from build123d import *

# Parameters (mm, degrees)
SKETCH1_W           = 50
SKETCH1_H           = 49.309999932
BOSS_EXTRUDE1_DEPTH = 22.098
SKETCH11_R          = 1.5875
CUT_EXTRUDE7_DEPTH  = 33.02
CUT_EXTRUDE8_DEPTH  = 2.54
BOSS_EXTRUDE5_DEPTH = 2.54
BOSS_EXTRUDE6_DEPTH = 7.5
SKETCH14_R          = 1.5875
SKETCH14_W          = 12.7
SKETCH14_H          = 12.7
CUT_EXTRUDE9_DEPTH  = 2.54
SKETCH20_W          = 6
SKETCH20_H          = 6.5
CUT_EXTRUDE13_DEPTH = 7.5
SKETCH22_R          = 2.667
BOSS_EXTRUDE7_DEPTH = 13.97999998
SKETCH24_R          = 1.5875
BOSS_EXTRUDE9_DEPTH = 2.54


with BuildPart() as part:
    # Sketch1 → Boss-Extrude1 (new body)
    with BuildSketch(Plane.XY):
        with Locations((0, 0.745000034)):
            Rectangle(SKETCH1_W, SKETCH1_H)
        Polygon((12.5, 47.050635095), (-12.5, 47.050635095), (-25, 25.4), (25, 25.4), align=None)
    extrude(amount=BOSS_EXTRUDE1_DEPTH)

    # Sketch11 → Cut-Extrude7 (cut)
    with BuildSketch(Plane.XY.offset(22.098)):
        with BuildLine():
            Line((-18.015, 22.179409051), (-19.92, 22.179409051))
            Line((-19.92, 22.179409051), (-19.92, -11.209999932))
            Line((-19.92, -11.209999932), (-18.65, -11.209999932))
            ThreePointArc((-18.65, -11.209999932), (-14.159871939, -13.069871871), (-12.3, -17.559999932))
            Line((-12.3, -17.559999932), (-12.3, -18.829999932))
            Line((-12.3, -18.829999932), (12.3, -18.829999932))
            Line((12.3, -18.829999932), (12.3, -17.559999932))
            ThreePointArc((12.3, -17.559999932), (14.159871939, -13.069871871), (18.65, -11.209999932))
            Line((18.65, -11.209999932), (19.92, -11.209999932))
            Line((19.92, -11.209999932), (19.92, 24.038818102))
            Line((19.92, 24.038818102), (18.060590949, 27.259409051))
            Line((18.060590949, 27.259409051), (9.567060633, 41.970635095))
            Line((9.567060633, 41.970635095), (-9.567060633, 41.970635095))
            Line((-9.567060633, 41.970635095), (-18.060590949, 27.259409051))
            Line((-18.060590949, 27.259409051), (-18.015, 27.259409051))
            ThreePointArc((-18.015, 27.259409051), (-12.935, 24.719409051), (-18.015, 22.179409051))
        make_face()
        with Locations((-16.11, 24.719409051)):
            Circle(SKETCH11_R)
        with Locations((16.11, -15.02)):
            Circle(SKETCH11_R)
        with Locations((-16.11, -15.02)):
            Circle(SKETCH11_R)
    extrude(amount=-CUT_EXTRUDE7_DEPTH, mode=Mode.SUBTRACT)

    # Sketch12 → Cut-Extrude8 (cut)
    with BuildSketch(Plane(origin=(0, 0, 0), x_dir=(-1, 0, 0), z_dir=(0, 0, -1))):
        Polygon((-22.46, 25.4), (-22.46, -21.369999932), (22.46, -21.369999932), (22.46, 25.4), (11.23, 44.850930569), (-11.23, 44.850930569), align=None)
    extrude(amount=-CUT_EXTRUDE8_DEPTH, mode=Mode.SUBTRACT)

    # Sketch13 → Boss-Extrude5 (add)
    with BuildSketch(Plane.XY.offset(22.098)):
        Polygon((-25, 25.4), (-25, -23.909999932), (25, -23.909999932), (25, 25.4), (12.5, 47.050635095), (-12.5, 47.050635095), align=None)
    extrude(amount=-BOSS_EXTRUDE5_DEPTH)

    # Sketch19 → Boss-Extrude6 (add)
    with BuildSketch(Plane(origin=(0, 0, 19.558), x_dir=(-1, 0, 0), z_dir=(0, 0, -1))):
        Polygon((-11.968279908, 28.961226002), (-11.968279908, 24.921226002), (-9.698279908, 24.921226002), (-9.698279908, 26.191226002), (-10.698279908, 26.191226002), (-10.698279908, 27.691226002), (-9.698279908, 27.691226002), (-9.698279908, 28.961226002), align=None)
        Polygon((4.601720092, 27.691226002), (4.601720092, 26.191226002), (3.601720092, 26.191226002), (3.601720092, 24.921226002), (5.871720092, 24.921226002), (5.871720092, 28.961226002), (3.601720092, 28.961226002), (3.601720092, 27.691226002), align=None)
    extrude(amount=BOSS_EXTRUDE6_DEPTH)

    # Sketch14 → Cut-Extrude9 (cut)
    with BuildSketch(Plane(origin=(0, 0, 19.558), x_dir=(-1, 0, 0), z_dir=(0, 0, -1))):
        with Locations((-10.16, 6.35)):
            Circle(SKETCH14_R)
        with Locations((10.16, 6.35)):
            Circle(SKETCH14_R)
        with Locations((10.16, -6.35)):
            Circle(SKETCH14_R)
        with Locations((-10.16, -6.35)):
            Circle(SKETCH14_R)
        Rectangle(SKETCH14_W, SKETCH14_H)
    extrude(amount=-CUT_EXTRUDE9_DEPTH, mode=Mode.SUBTRACT)

    # Sketch20 → Cut-Extrude13 (cut)
    with BuildSketch(Plane(origin=(0, 0, 19.558), x_dir=(-1, 0, 0), z_dir=(0, 0, -1))):
        with Locations((-0.698279908, 30.191226002)):
            Rectangle(SKETCH20_W, SKETCH20_H)
    extrude(amount=-CUT_EXTRUDE13_DEPTH, mode=Mode.SUBTRACT)

    # Sketch22 → Boss-Extrude7 (add)
    with BuildSketch(Plane.XY.offset(22.098)):
        with BuildLine():
            Line((26.155685571, 27.78125), (23.625184671, 27.78125))
            Line((23.625184671, 27.78125), (25, 25.4))
            Line((25, 25.4), (25, 23.33625))
            Line((25, 23.33625), (30.600685571, 23.33625))
            ThreePointArc((30.600685571, 23.33625), (33.743775214, 30.924339642), (26.155685571, 27.78125))
        make_face()
        with Locations((30.600685571, 27.78125)):
            Circle(SKETCH22_R, mode=Mode.SUBTRACT)
    extrude(amount=-BOSS_EXTRUDE7_DEPTH)

    # Sketch24 → Boss-Extrude9 (add)
    with BuildSketch(Plane(origin=(0, 0, 2.54), x_dir=(-1, 0, 0), z_dir=(0, 0, -1))):
        Polygon((11.23, 44.850930569), (-11.23, 44.850930569), (-22.46, 25.4), (-22.46, -21.369999932), (22.46, -21.369999932), (22.46, 25.4), align=None)
        with Locations(Location((16.11, -15.02, 0), (0, 0, 180))):
            Circle(SKETCH24_R, mode=Mode.SUBTRACT)
        with Locations(Location((16.11, 24.719409051, 0), (0, 0, 180))):
            Circle(SKETCH24_R, mode=Mode.SUBTRACT)
        with Locations(Location((-16.11, -15.02, 0), (0, 0, 180))):
            Circle(SKETCH24_R, mode=Mode.SUBTRACT)
        with BuildLine():
            Line((-19.92, 24.038818102), (-9.567060633, 41.970635095))
            Line((-9.567060633, 41.970635095), (9.567060633, 41.970635095))
            Line((9.567060633, 41.970635095), (18.060590949, 27.259409051))
            Line((18.060590949, 27.259409051), (18.015, 27.259409051))
            ThreePointArc((18.015, 27.259409051), (12.935, 24.719409051), (18.015, 22.179409051))
            Line((18.015, 22.179409051), (19.92, 22.179409051))
            Line((19.92, 22.179409051), (19.92, -11.209999932))
            Line((19.92, -11.209999932), (18.65, -11.209999932))
            ThreePointArc((18.65, -11.209999932), (14.159871939, -13.069871871), (12.3, -17.559999932))
            Line((12.3, -17.559999932), (12.3, -18.829999932))
            Line((12.3, -18.829999932), (-12.3, -18.829999932))
            Line((-12.3, -18.829999932), (-12.3, -17.559999932))
            ThreePointArc((-12.3, -17.559999932), (-14.159871939, -13.069871871), (-18.65, -11.209999932))
            Line((-18.65, -11.209999932), (-19.92, -11.209999932))
            Line((-19.92, -11.209999932), (-19.92, 24.038818102))
        make_face(mode=Mode.SUBTRACT)
    extrude(amount=BOSS_EXTRUDE9_DEPTH)


solid = part.part
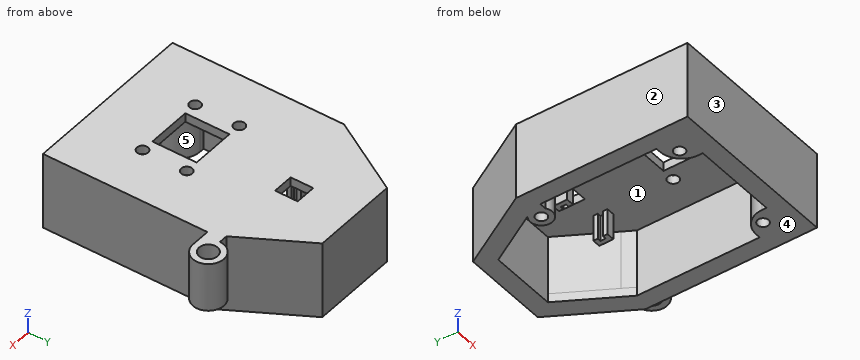
Work out the finished part from the listing and answer in its coordinate system (mm). Face numbers are marked on the shaded views. A direction names the side the tool comes from. Give positions to 0.01 mm unless a question says otherwise; leave off trailing zeros. Order: outer loops, then holes, each group sorted by start corner. A loop starts at its lowest first (then second) coordinate and runs counter-clockwise, first axis right, second up. Notation, with made-up numbers: (57, 26) -> (83, 26) arc R23 cw to (83, 39) -> close; hole circle Ø10 at (47, -17). An arc over 180 degrees is marked (long way). One line per item, written item: value.
Item 1: Find section B-B, the plane y = 18. Give the vertices of the cut face in (x, z), plus the area to 3 significant figures.
Answer sheet:
outline: (-25, 0) -> (-19.92, 0) -> (-19.92, 19.56) -> (19.92, 19.56) -> (19.92, 0) -> (25, 0) -> (25, 22.1) -> (-25, 22.1) -> close
area: 326 mm²
Item 2: Find section C-C, the plane z = 6.75. State how many separate pieces and enclosed holes the cut face has, plus the area to 3 significant figures.
Answer sheet:
separate pieces: 1
enclosed holes: 4
area: 1,150 mm²
Item 3: A tool of negligible diameter and unlimited length cuts with its end or side. For the marked faces 4 and 5, from which of +Z, -Z, +X, -X, +Y, -Y can it reach the whole face along a straight path? Write none if from no direction.
Answer sheet:
face 4: -Z, +X, -X, +Y, -Y
face 5: -Z
Item 4: Straight lines are drawn through the part: probe 1 along Y at (x, z) = (10.16, 20.55); probe 2 along X at (y, z) = (18.5, 10.5); probe 3 along Y at (x, z) = (-16.11, 10.5). For each, find the intervals that lie inside material, in ascending order.
Answer sheet:
probe 1: -23.91 to -7.94, -4.76 to 4.76, 7.94 to 47.05
probe 2: -25 to -19.92, 19.92 to 25
probe 3: -23.91 to -16.61, -13.43 to -11.74, 21.54 to 23.13, 26.31 to 27.89, 30.64 to 40.8
Item 5: Determine the mould class of the marked faces 1, 2 and 3 for opening direction X: released by +X, released by -X, zero draft, split by the parting line, or undercut.
Answer sheet:
face 1: undercut
face 2: released by -X
face 3: zero draft
Item 6: Flat-ended cylindrical pins translate along their axes: P1, Ø1, axis at x = 7.5, y = 25, coming from the -Z side; P2, Ø1.2, axis at y = 26.5, z = 14.5, coming from the -X side; P3, Ø2, axis at x = 25, z = 17.5, coming from the +Y side; P4, Ø1.4, axis at y = 28.5, z = 17, coming from the +X side. Find the tip coordinate at first contact, or state that the pin passes through.
Answer sheet:
P1: z = 19.56
P2: x = -24.71
P3: y = 27.78
P4: x = 35.05
Item 7: Find section A-A, the plane y = 3. Give the vertices of the cut face in (x, z).
Answer sheet:
outline: (-25, 0) -> (-19.92, 0) -> (-19.92, 19.56) -> (-6.35, 19.56) -> (-6.35, 22.1) -> (-25, 22.1) -> close; (6.35, 19.56) -> (19.92, 19.56) -> (19.92, 0) -> (25, 0) -> (25, 22.1) -> (6.35, 22.1) -> close
Item 8: Find section D-D, the plane x = -16.11. Give the vertices of the cut face in (y, z).
Answer sheet:
outline: (-23.91, 0) -> (-16.61, 0) -> (-16.61, 19.56) -> (-13.43, 19.56) -> (-13.43, 0) -> (-11.74, 0) -> (-11.74, 19.56) -> (21.54, 19.56) -> (21.54, 0) -> (23.13, 0) -> (23.13, 19.56) -> (26.31, 19.56) -> (26.31, 0) -> (27.89, 0) -> (27.89, 19.56) -> (30.64, 19.56) -> (30.64, 0) -> (40.8, 0) -> (40.8, 22.1) -> (-23.91, 22.1) -> close
